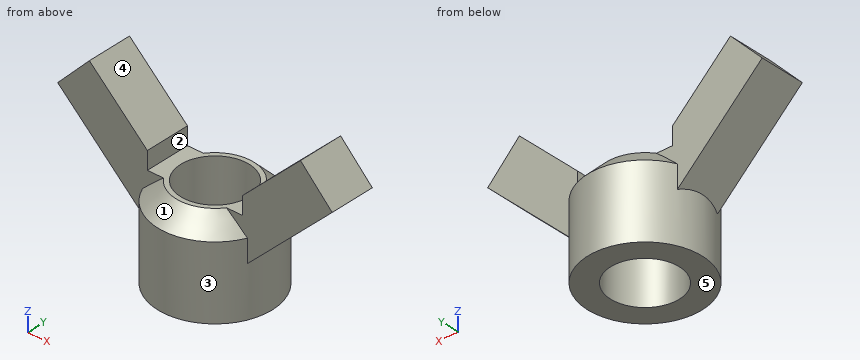
```python
from build123d import *

# Parameters (mm, degrees)
F1_DEPTH      = 3.175
F1_DEPTH_BACK = 3.175
F2_R          = 7.9375
F2_R_2        = 4.7625
F3_DEPTH      = 12.7
F4_T4_ANGLE   = 227.2280154593
F4_T9_ANGLE   = 227.2280154593


# Not quite as in the source:
# - a fillet or chamfer that OpenCascade refuses, or shapes differently, is made with other operations: its cross-section is extruded or revolved along the edge and cut away or added


with BuildPart() as f1:
    # F0 (on Front) → F1 (new body, two sides)
    with BuildSketch(Plane.XZ) as f1_sk:
        Polygon((-19.05, 18.3173076923), (-6.604, 6.35), (-6.604, 15.1592518354), (-14.6487596518, 22.8945976544), align=None)
    extrude(amount=F1_DEPTH)
    extrude(f1_sk.sketch, amount=-F1_DEPTH_BACK)



with BuildPart() as f1b:
    # F0 (on Front) → F1, piece 2 (new body, two sides)
    with BuildSketch(Plane.XZ) as f1_2_sk:
        Polygon((6.604, 15.1592518354), (6.604, 6.35), (19.05, 18.3173076923), (14.6487596518, 22.8945976544), align=None)
    extrude(amount=F1_DEPTH)
    extrude(f1_2_sk.sketch, amount=-F1_DEPTH_BACK)


with BuildPart() as f1_1:
    add(f1.part)

    add(f1b.part)  # F3 merges F1b
    # F2 (on Top) → F3 (join)
    with BuildSketch(Plane.XY):
        Circle(F2_R)
        Circle(F2_R_2, mode=Mode.SUBTRACT)
    extrude(amount=F3_DEPTH)

    # F4: chamfer of 2.54 on 2 edges, made by hand


with BuildPart() as f4_tool2:
    # F4_s3 → F4_t4 (revolve)
    with BuildSketch(Plane(origin=(0, 0, 0), x_dir=(0, 0, 1), z_dir=(0.4005730539, 0.9162648244, 0))):
        with BuildLine():
            Line((10.088157951, -8.009342049), (12.771842049, -5.325657951))
            Line((12.771842049, -5.325657951), (12.822642049, -5.325657951))
            ThreePointArc((12.822642049, -5.325657951), (12.7508, -6.6315789755), (12.7508, -7.9375))
            Line((12.7508, -7.9375), (12.7, -7.9883))
            ThreePointArc((12.7, -7.9883), (11.3940789755, -7.9883), (10.088157951, -8.060142049))
            Line((10.088157951, -8.060142049), (10.088157951, -8.009342049))
        make_face()
    revolve(axis=Axis((0, 0, 12.7), (0, 0, 1)), revolution_arc=F4_T4_ANGLE)

    split(bisect_by=Plane.XZ.offset(3.175), keep=Keep.TOP)


with BuildPart() as f1_2:
    add(f1_1.part)

    # F4_t1: cut F4_tool2
    add(f4_tool2.part, mode=Mode.SUBTRACT)


with BuildPart() as f4_tool7:
    # F4_s8 → F4_t9 (revolve)
    with BuildSketch(Plane(origin=(0, 0, 0), x_dir=(0, 0, 1), z_dir=(-0.4005730539, -0.9162648244, 0))):
        with BuildLine():
            Line((10.088157951, -8.009342049), (12.771842049, -5.325657951))
            Line((12.771842049, -5.325657951), (12.822642049, -5.325657951))
            ThreePointArc((12.822642049, -5.325657951), (12.7508, -6.6315789755), (12.7508, -7.9375))
            Line((12.7508, -7.9375), (12.7, -7.9883))
            ThreePointArc((12.7, -7.9883), (11.3940789755, -7.9883), (10.088157951, -8.060142049))
            Line((10.088157951, -8.060142049), (10.088157951, -8.009342049))
        make_face()
    revolve(axis=Axis((0, 0, 12.7), (0, 0, 1)), revolution_arc=F4_T9_ANGLE)

    split(bisect_by=Plane.XZ.offset(-3.175), keep=Keep.BOTTOM)


with BuildPart() as f1_3:
    add(f1_2.part)

    # F4_t6: cut F4_tool7
    add(f4_tool7.part, mode=Mode.SUBTRACT)


solid = f1_3.part
```
For this review, take the finished solid that the model builds, in its own axes (mm). Face numbers are marked on the shaded views. A direction names the side the tool comes from. Coordinates: 2 decimals unless noted, no trailing zeros. Order: outer loops, then holes, each group sorted by start corner. A loop starts at its lowest first (then second) coordinate and runs counter-clockwise, first axis right, second up. Notation, with made-up numbers: (89.5, 50) - (108.5, 50) arc R27 ccw to (108.5, 74) - close; hole circle Ø4 at (-18.75, 89). An arc over 180 degrees is marked (long way). Answer as a JSON object with one key per item and string values. Group by question number.
1. Clearance check with flat-ended pins moving along their axes: P1, Ø5.5, axis at x = 0, y = 0, coming from the -Z side; P2, Ø6, axis at x = -1.5, y = 6, coming from the +Z side; P3, Ø2, axis at y = -1, z = 14.5, coming from the +X side; P4, Ø4, axis at x = 12.5, y = -1.5, coming from the +Z side. State where each tip first meets the part, or that it passes through.
2. We need section D-D on y = -1.25. State the section outline as (x, z) points, then the cut area to 3 significant figures.
3. We need section B-B on y = 2. State the section outline as (x, z) points, then the cut area to 3 significant figures.
4. For probe 1 along Y at (x, z) = (0, 3.25); probe 2 along Z at (x, y) = (5, 2.75); probe 3 along Y at (x, z) = (14.5, 17.25) (3 decimals), list the stretches that pass through material, from the lowest coordinate up.
5. The part is to be moulded in two halves that separate along X. For the marked faces 3, 4 and 5, say which applies: pulls with the +X half, pulls with the -X half, needs draft (parallel to the pull), parting line crosses it, or undercut.
6. For the marked faces 1 and 2, list the 3-axis set-ups (+Z, -Z, +X, -X, +Y, -Y) from which the entire face can be reached by the end or side of a thin tool; tool diameter is ignored.
7. We need section C-C on z = 3.25. State the section outline as (x, y) points (1 decimal).
8. We need section A-A on x = 0. State the section outline as (y, z) points, then the cut area to 3 significant figures.
Final values:
{
 "1": {"P1": "through", "P2": "z = 12.7", "P3": "x = 16.12", "P4": "z = 22.75"},
 "2": {"outline": "(-19.05, 18.32) - (-7.84, 7.54) - (-7.84, 0) - (-4.6, 0) - (-4.6, 12.7) - (-6.6, 12.7) - (-6.6, 15.16) - (-14.65, 22.89) - close; (4.6, 0) - (7.84, 0) - (7.84, 7.54) - (19.05, 18.32) - (14.65, 22.89) - (6.6, 15.16) - (6.6, 12.7) - (4.6, 12.7) - close", "area": "249 mm²"},
 "3": {"outline": "(-19.05, 18.32) - (-7.68, 7.39) - (-7.68, 0) - (-4.32, 0) - (-4.32, 12.7) - (-6.6, 12.7) - (-6.6, 15.16) - (-14.65, 22.89) - close; (4.32, 0) - (7.68, 0) - (7.68, 7.39) - (19.05, 18.32) - (14.65, 22.89) - (6.6, 15.16) - (6.6, 12.7) - (4.32, 12.7) - close", "area": "253 mm²"},
 "4": {"probe 1": "-7.94 to -4.76, 4.76 to 7.94", "probe 2": "0 to 12.7", "probe 3": "-3.175 to 3.175"},
 "5": {"face 3": "parting line crosses it", "face 4": "undercut", "face 5": "needs draft"},
 "6": {"face 1": "+Z, -Y", "face 2": "+Z, +Y, -Y"},
 "7": {"outline": "circle Ø15.9 at (0, 0); hole circle Ø9.5 at (0, 0)"},
 "8": {"outline": "(-7.94, 0) - (-4.76, 0) - (-4.76, 12.7) - (-5.4, 12.7) - (-7.94, 10.16) - close; (4.76, 0) - (7.94, 0) - (7.94, 10.16) - (5.4, 12.7) - (4.76, 12.7) - close", "area": "74.2 mm²"}
}
